Autodesk Inventor part; units mm, degrees
ref_plane "YZ Plane" through (0, 0, 0) normal (1, 0, 0) x (0, 1, 0)
ref_plane "XZ Plane" through (0, 0, 0) normal (0, 1, 0) x (-1, 0, 0)
ref_plane "XY Plane" through (0, 0, 0) normal (0, 0, 1) x (1, 0, 0)
sketch "Sketch1" plane through (0, 0, 0) normal (0, 0, 1) x (1, 0, 0)
  line L0 (-0.2, 0.9842) -> (-0.2, 0.8)
  line L1 (-0.2, 0.8) -> (-0.5, 0.8)
  line L2 (-0.5, 0.8) -> (-0.5, 0)
  line L3 (-0.5, 0) -> (0.5, 0)
  line L4 (0.5, 0) -> (0.5, 0.8)
  line L5 (0.5, 0.8) -> (0.2, 0.8)
  line L6 (0.2, 0.8) -> (0.2, 0.9842)
  line L7 (0.2, 0.9842) -> (0.2, 2.3)
  line L8 (0.2, 2.3) -> (1.5, 2.3)
  line L9 (1.5, 2.3) -> (1.5, 5.8)
  line L10 (1.5, 5.8) -> (-1.5, 5.8)
  line L11 (-1.5, 5.8) -> (-1.5, 2.3)
  line L12 (-1.5, 2.3) -> (-0.2, 2.3)
  line L13 (-0.2, 0.9842) -> (-0.2, 2.3)
  line L14 (0, 5.8) -> (0, 0) construction
  line L15 (-0.2, 2.3) -> (0.2, 2.3)
  line L16 (0, 5.8) -> (0, 2.3)
  line L17 (0, 5.8) -> (3, 5.8)
  line L18 (4, 6.8) -> (4, 6.8)
  line L19 (3, 7.8) -> (0, 7.8)
  line L20 (0, 7.8) -> (0, 5.8)
  arc A0 (4, 6.8) -> (3, 7.8) centre (3, 6.8) ccw
  arc A1 (3, 5.8) -> (4, 6.8) centre (3, 6.8) ccw
  point P0 (4, 7.8)
  point P1 (4, 5.8)
  point P2 (4, 6.8)
  dimension "d0" = 0.4
  dimension "d1" = 3
  dimension "d2" = 1
  dimension "d3" = 0.8
  dimension "d4" = 1.5
  dimension "d5" = 3.5
  dimension "d12" = 2
  dimension "d13" = 1
  dimension "d14" = 1
  dimension "d15" = 3
extrude "Extrusion1" add sketch "Sketch1" along normal mid plane 3 contours L13 L15 L7 L6 L5 L4 L3 L2 L1 L0
revolve "Revolution1" add sketch "Sketch1" angle 360 about axis through (0, 5.8, 0) along (0, -1, 0) contours L16 L10 L9 L8 L15
sketch "Sketch2" plane through (-0.5, 0, 1.5) normal (0, -1, 0) x (1, 0, 0)
  circle A0 centre (0.5, -1.5) radius 1.5
  arc A1 (0.3, -0.0134) -> (0.3, -2.9866) centre (0.5, -1.5) ccw
  line L0 (0, -0.0858) -> (0, 0)
  line L1 (0, 0) -> (0.5, 0)
  line L2 (0, 0) -> (1, 0)
  line L3 (1, 0) -> (0.7, 0)
  line L4 (0.5, 0) -> (1, 0)
  line L5 (1, 0) -> (1, -0.0858)
  line L6 (0, -3) -> (0, 0)
  line L7 (0, -2.9142) -> (0, -3)
  line L8 (0.3, -3) -> (0.5, -3)
  line L9 (0, -3) -> (0.5, -3)
  line L10 (1, -3) -> (1, 0)
  line L11 (0.5, -3) -> (1, -3)
  line L12 (1, -3) -> (1, -2.9142)
  dimension "d9" = 3
extrude "Extrusion2" cut sketch "Sketch2" against normal up to surface (2.3 mm away) contours A0 L2 L5 | L10 L11 A0 | A0 L0 L1 | L8 L9 L6 A0
revolve "Revolution2" add sketch "Sketch1" angle 360 about axis through (0, 7.8, 0) along (0, -1, 0) contours L20 L19 A0 A1 L17 L10
properties part number "Taster_Top"
The listing builds one solid part. Answer for the finished solid, in the listing's coordinates (mm). A direction names the side the tool comes from. Coordinates: 2 decimals unless noted, no trailing zeros. Write each loop counter-clockwise with the first axis right and the second up, starting at its lowest first coordinate (ties: lowest second). Pieces come first, ordered by that corner, then holes. Notation, with made-up numbers: M 49,9.5 L 93,9.5 A23 cw 93,25.5 Z; hole C -31.5,-36.75 d11. An arc over 180 degrees is marked long. Put each result on its own line as item: value. Start each with the question number.
1. Consider line 1 (Y direction, x = -0.25, z = 0.5); line 2 (Y direction, x = 2.25, z = 0); line 3 (Z direction, x = 0.5, y = 3.25). Determine where each line is inside the solid, lowest interval first. Write a range as from..to.
2. Which of the six approach directions +Z, -Z, +X, -X, +Y, -Y give full straight-line access (tool end or side, diameter ignored) to faces 5 (the flat face through (1.3, 5.8, -1.3)), 6 (the flat face through (1, 2.3, 0)), 7 (the flat face through (-1, 2.3, 0)), 8 (the flat face through (0, 7.8, 0))?
3. A cutting plane is placed at A-A on z = 0. Write down the section's boundary in (x, y).
4. A cutting plane is placed at C-C on y = 3.25. Write down the section's boundary in (x, z).
5. A cutting plane is placed at D-D on y = 7.25. Write down the section's boundary in (x, z), then the cut area to 3 significant figures.
6. Flat-ended cylindrical pins translate along their axes: P1, Ø0.9, axis at y = 0.5, z = 0.5, coming from the +X side; P2, Ø1.2, axis at y = 1.5, z = -0.5, coming from the -X side; P3, Ø4, axis at x = -1, z = 1, coming from the -Y side; P4, Ø3, axis at x = 2.5, y = 6, coming from the +Z side. Find the tip coordinate at first contact, or state that the pin passes through.
7. A cutting plane is placed at B-B on x = 0. Write down the section's boundary in (y, z).
8. For a pull along Y with two mould halves and no side action, classify faces 1 (the flat face through (-0.2, 2, 0)), 2 (the flat face through (0, 0, 0)), 3 (the flat face through (0.2, 2, 0)), 4 (the cylindrical face through (-0.195, 4.229, -1.487)) as pulls with the +Y half, pulls with the -Y half, needs draft (parallel to the pull), parting line crosses it, or undercut.
Resolved:
1. line 1: y = 0..0.8, 2.3..7.8
1. line 2: y = 5.8..7.8
1. line 3: z = -1.41..1.41
2. face 5: -Y
2. face 6: +Z, -Z, +X
2. face 7: +Z, -Z, -X
2. face 8: +Z, -Z, +X, -X, +Y
3. outline: M -3,5.8 L -1.5,5.8 L -1.5,2.3 L -0.2,2.3 L -0.2,0.8 L -0.5,0.8 L -0.5,0 L 0.5,0 L 0.5,0.8 L 0.2,0.8 L 0.2,2.3 L 1.5,2.3 L 1.5,5.8 L 3,5.8 A1 ccw 3,7.8 L -3,7.8 A1 ccw Z
4. outline: C 0,0 d3
5. outline: C 0,0 d7.79
5. area: 47.6 mm2
6. P1: stops at x = 0.5
6. P2: stops at x = -0.2
6. P3: stops at y = 0
6. P4: stops at z = 3.82
7. outline: M 0,-1.5 L 5.8,-1.5 L 5.8,-3 A1 ccw 7.8,-3 L 7.8,3 A1 ccw 5.8,3 L 5.8,1.5 L 0,1.5 Z
8. face 1: undercut
8. face 2: pulls with the -Y half
8. face 3: undercut
8. face 4: needs draft
